```python
from build123d import *

# Parameters (mm, degrees)
BOSS_EXTRUDE1_DEPTH                               = 19.05
CSK_FOR_8_FLAT_HEAD_MACHINE_SCREW_100_D           = 4.9149
CSK_FOR_8_FLAT_HEAD_MACHINE_SCREW_100_CSINK_D     = 8.4328
CSK_FOR_8_FLAT_HEAD_MACHINE_SCREW_100_CSINK_ANGLE = 100


with BuildPart() as part:
    # Sketch1 → Boss-Extrude1 (new body)
    with BuildSketch(Plane.XY):
        Polygon((2683.51, 6983.72999014), (2683.51, 6641.741886848), (3140.71, 6826.4626773), (3140.71, 6983.72999014), align=None)
    extrude(amount=BOSS_EXTRUDE1_DEPTH)

    # CSK for #8 Flat Head Machine Screw (100)1 (through all)
    with Locations(Plane.YX):
        with Locations((6692.541891629, 2721.610000001), (6945.629994921, 2721.610000001), (6945.629994921, 3115.310000001), (6851.60701674, 3115.310000001)):
            CounterSinkHole(CSK_FOR_8_FLAT_HEAD_MACHINE_SCREW_100_D / 2, CSK_FOR_8_FLAT_HEAD_MACHINE_SCREW_100_CSINK_D / 2, counter_sink_angle=CSK_FOR_8_FLAT_HEAD_MACHINE_SCREW_100_CSINK_ANGLE)


solid = part.part
```
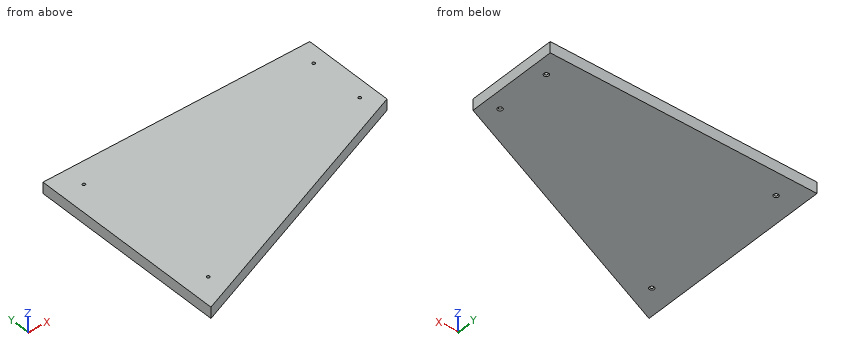
Geometry check sheet. Reference: the model listing, model coordinates, mm. Give positions to 0.01 mm unless a question says otherwise; leave off trailing zeros. Write each loop counter-clockwise with the first axis right and the second up, starting at its lowest first coordinate (ties: lowest second). Pieces come first, ordered by that corner, then holes.
1) Section check A-A, the plane z = 14.5. Record the boundary of the cut face in (x, y).
2) Material ranges on L1, parallel to X at y = 6946, z = 17.5; L2, parallel to X at y = 6944.5, z = 3.5; L3, parallel to Y at x = 2918, z = 17.25, recorded low to high.
3) Section check B-B, the plane x = 3043. Record the boundary of the cut face in (y, z), and give its area (3 significant figures).
4) Gauge pin test, flat ends, axial feed: pin 1 (6.5 mm diameter, centred on x = 3115.31, y = 6945.63, fed in from -Z); pin 2 (6 mm diameter, centred on x = 2877, z = 10, fed in from -Y); pin 3 (4 mm diameter, centred on x = 2721.61, y = 6692.54, fed in from +Z); pin 4 (8 mm diameter, centred on x = 3115.31, y = 6851.61, fed in from -Z). Record the tip position at first contact, or that the pin passes through.
5) Section check C-C, the plane y = 6707.5. Record the boundary of the cut face in (x, z), and give its area (3 significant figures).
Computed:
1. outline: (2683.51, 6641.74) - (3140.71, 6826.46) - (3140.71, 6983.73) - (2683.51, 6983.73) - close; hole circle Ø4.91 at (2721.61, 6692.54); hole circle Ø4.91 at (2721.61, 6945.63); hole circle Ø4.91 at (3115.31, 6851.61); hole circle Ø4.91 at (3115.31, 6945.63)
2. L1: x = 2683.51 to 2719.18, 2724.04 to 3112.88, 3117.74 to 3140.71
2. L2: x = 2683.51 to 2719.43, 2723.79 to 3113.13, 3117.49 to 3140.71
2. L3: y = 6736.48 to 6983.73
3. outline: (6786.99, 0) - (6983.73, 0) - (6983.73, 19.05) - (6786.99, 19.05) - close
3. area: 3,750 mm2
4. pin 1: stops at z = 0.81
4. pin 2: stops at y = 6718.7
4. pin 3: passes through
4. pin 4: stops at z = 0.18
5. outline: (2683.51, 0) - (2846.27, 0) - (2846.27, 19.05) - (2683.51, 19.05) - close
5. area: 3,100 mm2
